Read the model definition and answer for the solid it produces. Units are mm, in the model's axes. A direction names the side the tool comes from. Coordinates: 2 decimals unless noted, no trailing zeros. Loops run counter-clockwise (first coordinate to the right, second up) from the corner with the lowest first, then second, coordinate; pieces in that order, holes last. Notation, with made-up numbers: (-9, -23.5) -> (32, -23.5) arc R34 cw to (32, 13.5) -> close; hole circle Ø8 at (-10.75, -35.75). An arc over 180 degrees is marked (long way). Answer as a JSON object with one key per item and string values. Group by question number.
Q1. Straight lines are drawn through the part: line 1 along X through (y, z) = (6.25, 2); line 2 along Z through (x, y) = (0, 2.5); line 3 along Y through (x, z) = (21, 6.75). For each, find the intervals that lie inside material, in ascending order. Write a range as [from, to].
Q2. For faces 1 (the cylindrical face through (51.32, 4.58, 7.53)), 2 (the cylindrical face through (81.5, -0.5, 2.2)), 3 (the flat face through (41, 9, -2)), 4 (the flat face through (67.26, 4.58, -0.75)), 5 (the cylindrical face through (-9, 5, 0)), determine the directions among +Z, -Z, +X, -X, +Y, -Y from which every point of the face is accessible in a straight line to the end or side of a thin tool.
Q3. The part is cut by section B-B on x = 40. Write down the section's boundary in (y, z).
Q4. The part is cut by section C-C on y = 2.5. Write down the section's boundary in (x, z), and give its area (3 significant figures).
Q5. The part is cut by section A-A on z = 6.5. Write down the section's boundary in (x, y), and give its area (3 significant figures).
Q6. Each of these flat-tipped pins is pushed along its axis until it touches: P1, Ø0.5, axis at x = 63.5, y = -0.5, coming from the +Z side; P2, Ø0.8, axis at y = -0.5, z = -2, coming from the -X side; P3, Ø0.5, axis at x = 63, y = 9.5, coming from the +Z side. Where does it stop, or does it pass through?
Q7. Determine the mould class of faces 6 (the cylindrical face through (49.74, -0.49, -1.48)), 7 (the flat face through (41.3, 10, -8.7)), 8 (the cylindrical face through (90.797, 4.577, -7.859)) for opening direction X: released by +X, released by -X, zero draft, split by the parting line, or undercut.
Q8. The part is cut by section D-D on x = 66. Write down the section's boundary in (y, z), and give its area (3 significant figures).
from build123d import *

# Parameters (mm, degrees)
SKETCH1_R           = 4.75
BOSS_EXTRUDE1_DEPTH = 9
BOSS_EXTRUDE2_DEPTH = 1
BOSS_EXTRUDE3_DEPTH = 1


with BuildPart() as part:
    # Sketch1 → Boss-Extrude1 (new body)
    with BuildSketch(Plane(origin=(0, 0, 0), x_dir=(1, 0, 0), z_dir=(0, 1, 0))):
        with BuildLine():
            Line((55.857100089, 3.173260641), (78.357100089, -1.609261996))
            ThreePointArc((78.357100089, -1.609261996), (80.775815642, -2.888858783), (82.158770817, -5.25))
            ThreePointArc((82.158770817, -5.25), (87.630021462, -8.960148481), (92, -4))
            Line((92, -4), (92, 5))
            ThreePointArc((92, 5), (90.828427125, 7.828427125), (88, 9))
            Line((88, 9), (0, 9))
            ThreePointArc((0, 9), (-9, 0), (0, -9))
            Line((0, -9), (49.040217235, -9))
            ThreePointArc((49.040217235, -9), (51.302454571, -7.564087513), (50.965992035, -4.905825787))
            ThreePointArc((50.965992035, -4.905825787), (50.540307373, 0.871975682), (55.857100089, 3.173260641))
        make_face()
        Circle(SKETCH1_R, mode=Mode.SUBTRACT)
    extrude(amount=BOSS_EXTRUDE1_DEPTH)

    # Sketch2 → Boss-Extrude2 (add)
    with BuildSketch(Plane(origin=(0, 9, 0), x_dir=(1, 0, 0), z_dir=(0, 1, 0))):
        with BuildLine():
            Line((0, -9), (49.040217235, -9))
            ThreePointArc((49.040217235, -9), (51.302454571, -7.564087513), (50.965992035, -4.905825787))
            ThreePointArc((50.965992035, -4.905825787), (50.540307373, 0.871975682), (55.857100089, 3.173260641))
            Line((55.857100089, 3.173260641), (78.357100089, -1.609261996))
            ThreePointArc((78.357100089, -1.609261996), (80.775815642, -2.888858783), (82.158770817, -5.25))
            ThreePointArc((82.158770817, -5.25), (87.630021462, -8.960148481), (92, -4))
            Line((92, -4), (92, 5))
            ThreePointArc((92, 5), (90.828427125, 7.828427125), (88, 9))
            Line((88, 9), (0, 9))
            ThreePointArc((0, 9), (-9, 0), (0, -9))
        make_face()
        with BuildLine():
            Line((88, 8), (0, 8))
            ThreePointArc((0, 8), (-8, 0), (0, -8))
            Line((0, -8), (49.040217235, -8))
            ThreePointArc((49.040217235, -8), (50.397559636, -7.138452508), (50.195682115, -5.543495472))
            ThreePointArc((50.195682115, -5.543495472), (49.68486052, 1.389866291), (56.065011779, 4.151408242))
            Line((56.065011779, 4.151408242), (78.565011779, -0.631114396))
            ThreePointArc((78.565011779, -0.631114396), (81.467470443, -2.166630539), (83.127016654, -5))
            ThreePointArc((83.127016654, -5), (87.50401717, -7.968118785), (91, -4))
            Line((91, -4), (91, 5))
            ThreePointArc((91, 5), (90.121320344, 7.121320344), (88, 8))
        make_face(mode=Mode.SUBTRACT)
    extrude(amount=BOSS_EXTRUDE2_DEPTH)

    # Sketch3 → Boss-Extrude3 (add)
    with BuildSketch(Plane.XZ):
        with BuildLine():
            Line((0, -9), (88, -9))
            ThreePointArc((88, -9), (90.828427125, -7.828427125), (92, -5))
            Line((92, -5), (92, 4))
            ThreePointArc((92, 4), (87.630021462, 8.960148481), (82.158770817, 5.25))
            ThreePointArc((82.158770817, 5.25), (80.775815642, 2.888858783), (78.357100089, 1.609261996))
            Line((78.357100089, 1.609261996), (55.857100089, -3.173260641))
            ThreePointArc((55.857100089, -3.173260641), (50.540307373, -0.871975682), (50.965992035, 4.905825787))
            ThreePointArc((50.965992035, 4.905825787), (51.302454571, 7.564087513), (49.040217235, 9))
            Line((49.040217235, 9), (0, 9))
            ThreePointArc((0, 9), (-9, 0), (0, -9))
        make_face()
        with BuildLine():
            Line((49.040217235, 8), (0, 8))
            ThreePointArc((0, 8), (-8, 0), (0, -8))
            Line((0, -8), (88, -8))
            ThreePointArc((88, -8), (90.121320344, -7.121320344), (91, -5))
            Line((91, -5), (91, 4))
            ThreePointArc((91, 4), (87.50401717, 7.968118785), (83.127016654, 5))
            ThreePointArc((83.127016654, 5), (81.467470443, 2.166630539), (78.565011779, 0.631114396))
            Line((78.565011779, 0.631114396), (56.065011779, -4.151408242))
            ThreePointArc((56.065011779, -4.151408242), (49.68486052, -1.389866291), (50.195682115, 5.543495472))
            ThreePointArc((50.195682115, 5.543495472), (50.397559636, 7.138452508), (49.040217235, 8))
        make_face(mode=Mode.SUBTRACT)
    extrude(amount=BOSS_EXTRUDE3_DEPTH)


solid = part.part
Final values:
{
 "1": {"line 1": "x = [-8.77, -4.31], [4.31, 49.83], [79.5, 92]", "line 2": "z = [-9, -4.75], [4.75, 9]", "line 3": "y = [0, 9]"},
 "2": {"face 1": "+Y, -Y", "face 2": "-Y", "face 3": "+Y", "face 4": "+Z, +Y, -Y", "face 5": "-X, +Y, -Y"},
 "3": {"outline": "(-1, -9) -> (10, -9) -> (10, -8) -> (9, -8) -> (9, 8) -> (10, 8) -> (10, 9) -> (-1, 9) -> (-1, 8) -> (0, 8) -> (0, -8) -> (-1, -8) -> close"},
 "4": {"outline": "(0, -9) -> (88, -9) arc R4 ccw to (92, -5) -> (92, 4) arc R5 ccw to (82.16, 5.25) arc R5 cw to (78.36, 1.61) -> (55.86, -3.17) arc R5 cw to (50.97, 4.91) arc R2.5 ccw to (49.04, 9) -> (0, 9) arc R9 ccw to start; hole circle Ø9.5 at (0, 0)", "area": "1,390 mm2"},
 "5": {"outline": "(-6.22, -1) -> (-4.66, -1) -> (-4.66, 0) -> (50.54, 0) -> (50.54, -1) -> (51.54, -1) -> (51.54, 10) -> (50.54, 10) -> (50.54, 9) -> (-4.66, 9) -> (-4.66, 10) -> (-6.22, 10) -> close; (82.67, -1) -> (83.88, -1) -> (83.88, 0) -> (90.12, 0) -> (90.12, -1) -> (91.33, -1) -> (91.33, 10) -> (90.12, 10) -> (90.12, 9) -> (83.88, 9) -> (83.88, 10) -> (82.67, 10) -> close", "area": "608 mm2"},
 "6": {"P1": "stops at z = -1.5", "P2": "stops at x = -8.86", "P3": "stops at z = -1.6"},
 "7": {"face 6": "undercut", "face 7": "zero draft", "face 8": "released by +X"},
 "8": {"outline": "(-1, -9) -> (10, -9) -> (10, -8) -> (9, -8) -> (9, -2.04) -> (10, -2.04) -> (10, -1.02) -> (-1, -1.02) -> (-1, -2.04) -> (0, -2.04) -> (0, -8) -> (-1, -8) -> close", "area": "75.9 mm2"}
}
